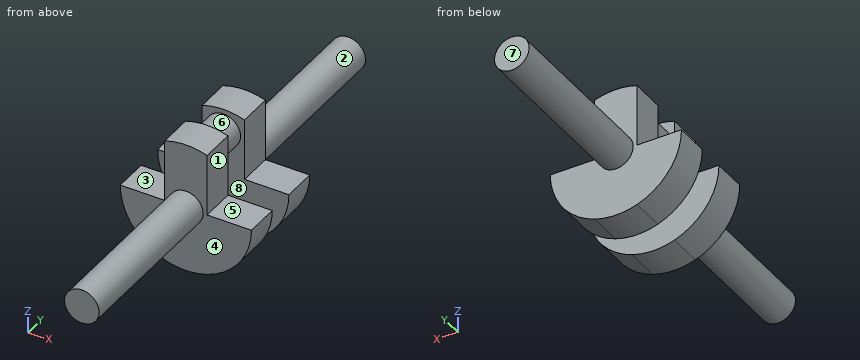
```python
from build123d import *

# Parameters (mm, degrees)
F1_DEPTH = 2.5
F2_R     = 2.5
F4_DEPTH = 14
F5_R     = 2.5
F6_DEPTH = 30
F7_R     = 2.5
F8_DEPTH = 30


# Not quite as in the source:
# - a feature names something its author has since deleted; it is built from what else it names


with BuildPart() as f1:
    # F0 (on Front) → F1 (new body, symmetric)
    with BuildSketch(Plane.XZ):
        with BuildLine():
            ThreePointArc((-3.0750329511, -8.9885578571), (0, -9.5), (3.0750329511, -8.9885578571))
            Line((3.0750329511, -8.9885578571), (3.0750329511, 0))
            Line((3.0750329511, 0), (3.0750329511, 8.9885578571))
            ThreePointArc((3.0750329511, 8.9885578571), (0, 9.5), (-3.0750329511, 8.9885578571))
            Line((-3.0750329511, 8.9885578571), (-3.0750329511, 0))
            Line((-3.0750329511, 0), (-3.0750329511, -8.9885578571))
        make_face()
        with BuildLine():
            ThreePointArc((-9.5, 0), (-7.7286096109, -5.5243636269), (-3.0750329511, -8.9885578571))
            Line((-3.0750329511, -8.9885578571), (-3.0750329511, 0))
            Line((-3.0750329511, 0), (-9.5, 0))
        make_face()
        with BuildLine():
            Line((3.0750329511, 0), (3.0750329511, -8.9885578571))
            ThreePointArc((3.0750329511, -8.9885578571), (7.7286096109, -5.5243636269), (9.5, 0))
            Line((9.5, 0), (3.0750329511, 0))
        make_face()
    extrude(amount=F1_DEPTH, both=True)


with BuildPart() as f3_1:
    # F3: copy of F1
    add(f1.part.moved(Location((0, 9, 0))))


with BuildPart() as f1_1:
    add(f1.part)

    add(f3_1.part)  # F4 merges F3_1
    # F2 (on face) → F4 (join, through all)
    with BuildSketch(Plane.XZ.offset(2.5)):
        with Locations((0, 6.3)):
            Circle(F2_R)
    extrude(amount=-F4_DEPTH)

    # F5 (on face) → F6 (join)
    with BuildSketch(Plane(origin=(0, 2.5, 0), x_dir=(-1, 0, 0), z_dir=(0, 1, 0))):
        Circle(F5_R)
    extrude(amount=-F6_DEPTH)

    # F7 (on face) → F8 (join)
    with BuildSketch(Plane.XZ.offset(-6.5)):
        Circle(F7_R)
    extrude(amount=-F8_DEPTH)


solid = f1_1.part
```
The listing builds one solid part. Answer for the finished solid, in the listing's coordinates (mm). Face numbers are marked on the shaded views. A direction names the side the tool comes from. Coordinates: 2 decimals unless noted, no trailing zeros. Write each loop counter-clockwise with the first axis right and the second up, starting at its lowest first coordinate (ties: lowest second). Pieces come first, ordered by that corner, then holes. Notation, with made-up numbers: (37.5, 1) - (79.5, 1) arc R18 ccw to (79.5, 8) - close; hole circle Ø4 at (-14.5, 66.5). An arc over 180 degrees is marked (long way). Return JSON: item names as keys, results as strings. Group by question number.
1. Straight lines are drawn through the part: L1, parallel to Y at x = 6.5, z = -2; L2, parallel to Y at x = 0.25, z = 6.5; L3, parallel to X at y = 1.5, z = 0.25. For each, find the intervals that lie inside material, in ascending order.
2. A cutting plane is placed at C-C, the plane z = 6.3. Determine the outline of the cut face in (x, y), plus the area to 3 significant figures.
3. A cutting plane is placed at D-D, the plane y = -7. Determine the outline of the cut face in (x, z).
4. A cutting plane is placed at A-A, the plane z = 0.75. Determine the outline of the cut face in (x, y), plus the area to 3 significant figures.
5. A cutting plane is placed at B-B, the plane x = -6. Determine the outline of the cut face in (y, z).
6. Determine the mould class of the marked faces 5, 6, 7 and 8 for opening direction Y: released by +Y, released by -Y, zero draft, split by the parting line, or undercut.
7. Given pin 1 (3 mm diameter, centred on x = 7.5, z = -7, fed in from -Y); pin 2 (6 mm diameter, centred on x = -2.5, z = 6, fed in from +Y); pin 3 (8 mm diameter, centred on x = -3.5, y = 25.5, fed in from -Z), each flat-ended and moving along its own axis, determine where each tip first touches the part or whether it passes through.
8. Which of the six approach directions +Z, -Z, +X, -X, +Y, -Y give full straight-line access (tool end or side, diameter ignored) to the marked faces 1, 2, 3 and 4?
Ans:
{
 "1": {"L1": "-2.5 to 2.5, 6.5 to 11.5", "L2": "-2.5 to 11.5", "L3": "-3.08 to 3.08"},
 "2": {"outline": "(-3.08, -2.5) - (3.08, -2.5) - (3.08, 2.5) - (2.5, 2.5) - (2.5, 6.5) - (3.08, 6.5) - (3.08, 11.5) - (-3.08, 11.5) - (-3.08, 6.5) - (-2.5, 6.5) - (-2.5, 2.5) - (-3.08, 2.5) - close", "area": "81.5 mm²"},
 "3": {"outline": "circle Ø5 at (0, 0)"},
 "4": {"outline": "(-3.08, -2.5) - (-2.38, -2.5) - (-2.38, -27.5) - (2.38, -27.5) - (2.38, -2.5) - (3.08, -2.5) - (3.08, 2.5) - (-3.08, 2.5) - close; (-3.08, 6.5) - (3.08, 6.5) - (3.08, 11.5) - (2.38, 11.5) - (2.38, 36.5) - (-2.38, 36.5) - (-2.38, 11.5) - (-3.08, 11.5) - close", "area": "300 mm²"},
 "5": {"outline": "(-2.5, -7.37) - (2.5, -7.37) - (2.5, 0) - (-2.5, 0) - close; (6.5, -7.37) - (11.5, -7.37) - (11.5, 0) - (6.5, 0) - close"},
 "6": {"face 5": "zero draft", "face 6": "undercut", "face 7": "released by +Y", "face 8": "undercut"},
 "7": {"pin 1": "y = -2.5", "pin 2": "y = 11.5", "pin 3": "z = -2.5"},
 "8": {"face 1": "+Z, +X, +Y, -Y", "face 2": "+Y", "face 3": "+Z, -X, +Y, -Y", "face 4": "-Y"}
}
